Geometry check sheet. Reference: the model listing, model coordinates, mm. A direction names the side the tool comes from. Give positions to 0.01 mm unless a question says otherwise; leave off trailing zeros. Loops run counter-clockwise (first coordinate to the right, second up) from the corner with the lowest first, then second, coordinate; pieces in that order, holes last.
1. Cross-section at B-B, the plane y = 47. Record the cut outline in (x, z), plus the area to 3 significant figures.
2. Material ranges on L1, parallel to X at y = 2.75, z = 50; L2, parallel to Z at x = -8, y = 51.5; L3, parallel to Y at x = 5, z = 17, recorded low to high.
3. Release check for a two-part mould opening along Z. For faces 4 (the flat face through (16.4, 10, 68.3)), 5 (the flat face through (-26.599, 4.93, 65.714)), 6 (the cylindrical face through (-37.197, 4.93, 42.228)) record: +Z half, -Z half, draft (parallel to the pull), parting line (faces both ways), or undercut.
4. Go/stop test with flat-tipped pins: pin 1 Ø3 at (y, z) = (41, -3) entering from -X; pin 2 Ø4 at (x, y) = (-1, 62.5) entering from +Z; pin 3 Ø1 at (x, z) = (0.5, 21) entering from +Y. Record where each tip stops, or that it passes through.
5. Cross-section at A-A, the plane z = 50. Record the cut outline in (x, y).
6. Tool access check on faces 1 (the flat face through (-11, 42, 0)), 2 (the cylindrical face through (0, 18, -5)), 3 (the flat face through (-29.314, 4.93, 60.359)). Record the directions out of +Z, -Z, +X, -X, +Y, -Y that give a thin tool (end or side, any length) a straight path to the whole face; none if there is none.
7. Cross-section at D-D, the plane y = 5.5. Record the cut outline in (x, z), plus the area to 3 significant figures.
from build123d import *

# Parameters (mm, degrees)
SKETCH1_W           = 50
SKETCH1_H           = 10
SKETCH1_R           = 7.5
BOSS_EXTRUDE1_DEPTH = 10
SKETCH1_3_W         = 50
SKETCH1_3_H         = 10
BOSS_EXTRUDE2_DEPTH = 75
CUT_EXTRUDE1_DEPTH  = 10
FILLET1_R           = 25


with BuildPart() as part:
    # Sketch1 → Boss-Extrude1 (new body)
    # profile 1 of 3: a face of its own
    with BuildSketch(Plane(origin=(0, 0, 0), x_dir=(1, 0, 0), z_dir=(0, 1, 0))):
        with BuildLine():
            Line((25, -17.151864589), (25, 0))
            Line((25, 0), (-25, 0))
            Line((-25, 0), (-25, -17.151864589))
            ThreePointArc((-25, -17.151864589), (-25.701702665, -20.83176495), (-27.708333333, -23.995226133))
            ThreePointArc((-27.708333333, -23.995226133), (0, -12), (27.708333333, -23.995226133))
            ThreePointArc((27.708333333, -23.995226133), (25.701702665, -20.83176495), (25, -17.151864589))
        make_face()
    # profile 2 of 3: a face of its own
    with BuildSketch(Plane(origin=(0, 0, 0), x_dir=(1, 0, 0), z_dir=(0, 1, 0))):
        with Locations((0, 5)):
            Rectangle(SKETCH1_W, SKETCH1_H)
    # profile 3 of 3: a face of its own
    with BuildSketch(Plane(origin=(0, 0, 0), x_dir=(1, 0, 0), z_dir=(0, 1, 0))):
        with BuildLine():
            ThreePointArc((35.600057015, -63.29044546), (37.256095308, -42.517796957), (27.708333333, -23.995226133))
            ThreePointArc((27.708333333, -23.995226133), (0, -12), (-27.708333333, -23.995226133))
            ThreePointArc((-27.708333333, -23.995226133), (-37.256095308, -42.517796957), (-35.600057015, -63.29044546))
            Line((-35.600057015, -63.29044546), (-22.848639927, -57.34436202))
            ThreePointArc((-22.848639927, -57.34436202), (21.751386889, -39.857161718), (-20.312930357, -62.782208742))
            Line((-20.312930357, -62.782208742), (-33.064347445, -68.728292182))
            ThreePointArc((-33.064347445, -68.728292182), (-31.119955968, -71.807070885), (-28.889805354, -74.685606061))
            ThreePointArc((-28.889805354, -74.685606061), (-21.739686255, -85.712027428), (-17.709540124, -98.220588235))
            ThreePointArc((-17.709540124, -98.220588235), (0, -113), (17.709540124, -98.220588235))
            ThreePointArc((17.709540124, -98.220588235), (21.739686255, -85.712027428), (28.889805354, -74.685606061))
            ThreePointArc((28.889805354, -74.685606061), (31.119955968, -71.807070885), (33.064347445, -68.728292182))
            ThreePointArc((33.064347445, -68.728292182), (34.439695907, -66.059493946), (35.600057015, -63.29044546))
        make_face()
        with Locations(Location((0, -95, 0), (0, 0, 270))):
            Circle(SKETCH1_R, mode=Mode.SUBTRACT)
    extrude(amount=BOSS_EXTRUDE1_DEPTH)

    # Sketch1<3> → Boss-Extrude2 (add)
    with BuildSketch(Plane(origin=(0, 0, 0), x_dir=(1, 0, 0), z_dir=(0, 1, 0))):
        with Locations((0, 5)):
            Rectangle(SKETCH1_3_W, SKETCH1_3_H)
    extrude(amount=BOSS_EXTRUDE2_DEPTH)

    # Sketch2 → Cut-Extrude1 (cut)
    with BuildSketch(Plane.XY):
        with BuildLine():
            Line((7, 50), (7, 25))
            ThreePointArc((7, 25), (0, 18), (-7, 25))
            Line((-7, 25), (-7, 50))
            ThreePointArc((-7, 50), (0, 57), (7, 50))
        make_face()
    extrude(amount=-CUT_EXTRUDE1_DEPTH, mode=Mode.SUBTRACT)

    # Fillet1
    fillet1_edges = [part.edges().sort_by_distance(p)[0] for p in [
        (-25, 75, -5),
        (25, 75, -5),
    ]]
    fillet(fillet1_edges, radius=FILLET1_R - 0.0001)  # a hair under: the kernel refuses the full size


solid = part.part
Result:
1. outline: (-25, -10) - (-7, -10) - (-7, 0) - (-25, 0) - close; (7, -10) - (25, -10) - (25, 0) - (7, 0) - close
1. area: 360 mm2
2. L1: x = -38 to -24, 24 to 38
2. L2: z = -10 to 0
2. L3: y = 0 to 10
3. face 4: draft
3. face 5: undercut
3. face 6: parting line
4. pin 1: stops at x = -25
4. pin 2: stops at z = 0
4. pin 3: stops at y = 10
5. outline: (-38, 0) - (-24, 0) - (-24, 10) - (-38, 10) - close; (24, 0) - (38, 0) - (38, 10) - (24, 10) - close
6. face 1: +Z, +X, -X, +Y
6. face 2: +Z, -Z
6. face 3: +Y, -Y
7. outline: (-35.6, 63.29) arc R38 ccw to (-27.71, 24) arc R10 cw to (-25, 17.15) - (-25, -10) - (25, -10) - (25, 17.15) arc R10 cw to (27.71, 24) arc R38 ccw to (28.89, 74.69) arc R50 cw to (17.71, 98.22) arc R18 ccw to (-17.71, 98.22) arc R50 cw to (-28.89, 74.69) arc R38 ccw to (-33.06, 68.73) - (-20.31, 62.78) arc R24 cw (long way) to (-22.85, 57.34) - close; hole circle Ø15 at (0, 95)
7. area: 4,610 mm2
